from build123d import *

# Parameters (mm, degrees)
EXTRUDE_1_DEPTH          = 45
SKETCH_2_R               = 17.5
CUT_EXTRUDE_1_DEPTH      = 40
SKETCH_3_R               = 14
CUT_EXTRUDE_2_DEPTH      = 63.596505494
CUT_EXTRUDE_3_DEPTH      = 10
CUT_EXTRUDE_3_DEPTH_BACK = 14
SKETCH_4_R               = 1.7
SKETCH_5_R               = 3
CUT_EXTRUDE_4_DEPTH      = 71.888257138
SKETCH_6_R               = 5
CUT_EXTRUDE_5_DEPTH      = 5
CUT_EXTRUDE_6_DEPTH      = 84.820179551


with BuildPart() as part:
    # Эскиз1 → Бобышка-Вытянуть1 (new body)
    with BuildSketch(Plane(origin=(0, 0, 0), x_dir=(1, 0, 0), z_dir=(0, 1, 0))):
        Polygon((-21.15, 21.15), (21.15, 21.15), (41.15, 21.15), (41.15, 11.15), (25, 11.15), (25, -25), (-25, -25), (-25, 11.15), (-41.15, 11.15), (-41.15, 21.15), align=None)
    extrude(amount=EXTRUDE_1_DEPTH)

    # Эскиз2 → Вырез-Вытянуть1 (cut)
    with BuildSketch(Plane.XZ):
        with Locations(Location((0, 0, 0), (0, 0, 270))):
            Circle(SKETCH_2_R)
    extrude(amount=-CUT_EXTRUDE_1_DEPTH, mode=Mode.SUBTRACT)

    # Эскиз3 → Вырез-Вытянуть2 (cut, through all)
    with BuildSketch(Plane.XZ.offset(-40)):
        with Locations(Location((0, 0, 0), (0, 0, 270))):
            Circle(SKETCH_3_R)
    extrude(amount=-CUT_EXTRUDE_2_DEPTH, mode=Mode.SUBTRACT)

    # Эскиз4 → Вырез-Вытянуть3 (cut, two sides: drawn at the far end of the back side and taken through both)
    with BuildSketch(Plane.XZ.offset(-40).offset(-CUT_EXTRUDE_3_DEPTH_BACK)):
        with Locations(Location((-12.374368671, -12.374368671, 0), (0, 0, 270))):
            Circle(SKETCH_4_R)
        with Locations(Location((12.374368671, -12.374368671, 0), (0, 0, 270))):
            Circle(SKETCH_4_R)
        with Locations(Location((12.374368671, 12.374368671, 0), (0, 0, 270))):
            Circle(SKETCH_4_R)
        with Locations(Location((-12.374368671, 12.374368671, 0), (0, 0, 270))):
            Circle(SKETCH_4_R)
    extrude(amount=CUT_EXTRUDE_3_DEPTH + CUT_EXTRUDE_3_DEPTH_BACK, mode=Mode.SUBTRACT)

    # Эскиз5 → Вырез-Вытянуть4 (cut, through all)
    with BuildSketch(Plane.XY.offset(-11.15)):
        with Locations((-33.075, 22.5)):
            Circle(SKETCH_5_R)
        with Locations((33.075, 22.5)):
            Circle(SKETCH_5_R)
    extrude(amount=-CUT_EXTRUDE_4_DEPTH, mode=Mode.SUBTRACT)

    # Эскиз6 → Вырез-Вытянуть5 (cut)
    with BuildSketch(Plane.XY.offset(-11.15)):
        with Locations((-33.075, 22.5)):
            Circle(SKETCH_6_R)
        with Locations((33.075, 22.5)):
            Circle(SKETCH_6_R)
    extrude(amount=-CUT_EXTRUDE_5_DEPTH, mode=Mode.SUBTRACT)

    # Эскиз7 → Вырез-Вытянуть6 (cut, through all)
    with BuildSketch(Plane(origin=(25, 0, 0), x_dir=(0, 0, -1), z_dir=(1, 0, 0))):
        Polygon((-25, 40), (11.15, 0), (-25, 0), align=None)
    extrude(amount=-CUT_EXTRUDE_6_DEPTH, mode=Mode.SUBTRACT)


solid = part.part
Work out the finished part from the listing and answer in its coordinate system (mm). A direction names the side the tool comes from. Coordinates: 2 decimals unless noted, no trailing zeros. Write each loop counter-clockwise with the first axis right and the second up, starting at its lowest first coordinate (ties: lowest second). Pieces come first, ordered by that corner, then holes.
1. The part is cut by section B-B, the plane z = 1.5. Write down the section's boundary in (x, y), and give its area (3 significant figures).
Results list:
outline: (-25, 14) - (-17.44, 14) - (-17.44, 40) - (-13.92, 40) - (-13.92, 45) - (-25, 45) - close; (13.92, 40) - (17.44, 40) - (17.44, 14) - (25, 14) - (25, 45) - (13.92, 45) - close
area: 504 mm2
2. The part is cut by section C-C, the plane y = 32.5. Write down the section's boundary in (x, z).
Results list:
outline: (-41.15, -21.15) - (41.15, -21.15) - (41.15, -11.15) - (25, -11.15) - (25, 18.22) - (-25, 18.22) - (-25, -11.15) - (-41.15, -11.15) - close; hole (-13.52, -11.12) arc R1.7 ccw (long way) to (-11.12, -13.52) arc R17.5 ccw to (11.12, -13.52) arc R1.7 ccw (long way) to (13.52, -11.12) arc R17.5 ccw to (13.52, 11.12) arc R1.7 ccw (long way) to (11.12, 13.52) arc R17.5 ccw to (-11.12, 13.52) arc R1.7 ccw (long way) to (-13.52, 11.12) arc R17.5 ccw to start
3. The part is cut by section A-A, the plane x = 4. Write down the section's boundary in (y, z), and give its area (3 significant figures).
Results list:
outline: (0, -21.15) - (45, -21.15) - (45, -13.42) - (40, -13.42) - (40, -17.04) - (0, -17.04) - close; (31.19, 17.04) - (40, 17.04) - (40, 13.42) - (45, 13.42) - (45, 25) - (40, 25) - close
area: 296 mm2
4. Flat-ended cylindrical pins translate along their axes: pin 1 (5 mm diameter, centred on x = -10.5, z = -6.5, fed in from -Y); pin 2 (7 mm diameter, centred on x = -33.075, y = 22.5, fed in from +Z); pin 3 (8 mm diameter, centred on x = 33, y = 24, fed in from +Z). Find the tip coordinate at first contact, or state that the pin passes through.
Results list:
pin 1: stops at y = 40
pin 2: stops at z = -16.15
pin 3: stops at z = -11.15
5. Consider line 1 along Y through (x, z) = (5, -13.5); line 2 along X through (y, z) = (34, 3.5); line 3 along Z through (x, y) = (-29, 38.5). Determine where each line is inside the solid, lowest interval first.
Results list:
line 1: y = 40 to 45
line 2: x = -25 to -17.15, 17.15 to 25
line 3: z = -21.15 to -11.15
6. For faces 1 (the flat face through (13, 30, 13)), 2 (the cylindrical face through (-28.46, 20.58, -13.62)), 3 (the flat face through (-25, 27, 3)), determine the directions among +Z, -Z, +X, -X, +Y, -Y from which every point of the face is accessible in a straight line to the end or side of a thin tool.
Results list:
face 1: +Y
face 2: +Z
face 3: +Z, -X, +Y, -Y
7. The part is cut by section D-D, the plane y = 22.5. Write down the section's boundary in (x, z) (3 decimals), and give its area (3 significant figures).
Results list:
outline: (-41.15, -21.15) - (-36.075, -21.15) - (-36.075, -16.15) - (-38.075, -16.15) - (-38.075, -11.15) - (-41.15, -11.15) - close; (-30.075, -21.15) - (30.075, -21.15) - (30.075, -16.15) - (28.075, -16.15) - (28.075, -11.15) - (25, -11.15) - (25, 9.184) - (14.896, 9.184) arc R17.5 cw (long way) to (-14.896, 9.184) - (-25, 9.184) - (-25, -11.15) - (-28.075, -11.15) - (-28.075, -16.15) - (-30.075, -16.15) - close; (36.075, -21.15) - (41.15, -21.15) - (41.15, -11.15) - (38.075, -11.15) - (38.075, -16.15) - (36.075, -16.15) - close
area: 893 mm2
8. For a pull along Z with two mould halves and no side action, classify faces 4 (the cylindrical face through (-30.304, 21.351, -18.615)), 5 (the flat face through (-13, 30, 13)), 6 (the flat face through (33, 17, -11.15)) as +Z half, -Z half, draft (parallel to the pull), parting line (faces both ways), or undercut.
Results list:
face 4: draft
face 5: undercut
face 6: +Z half
